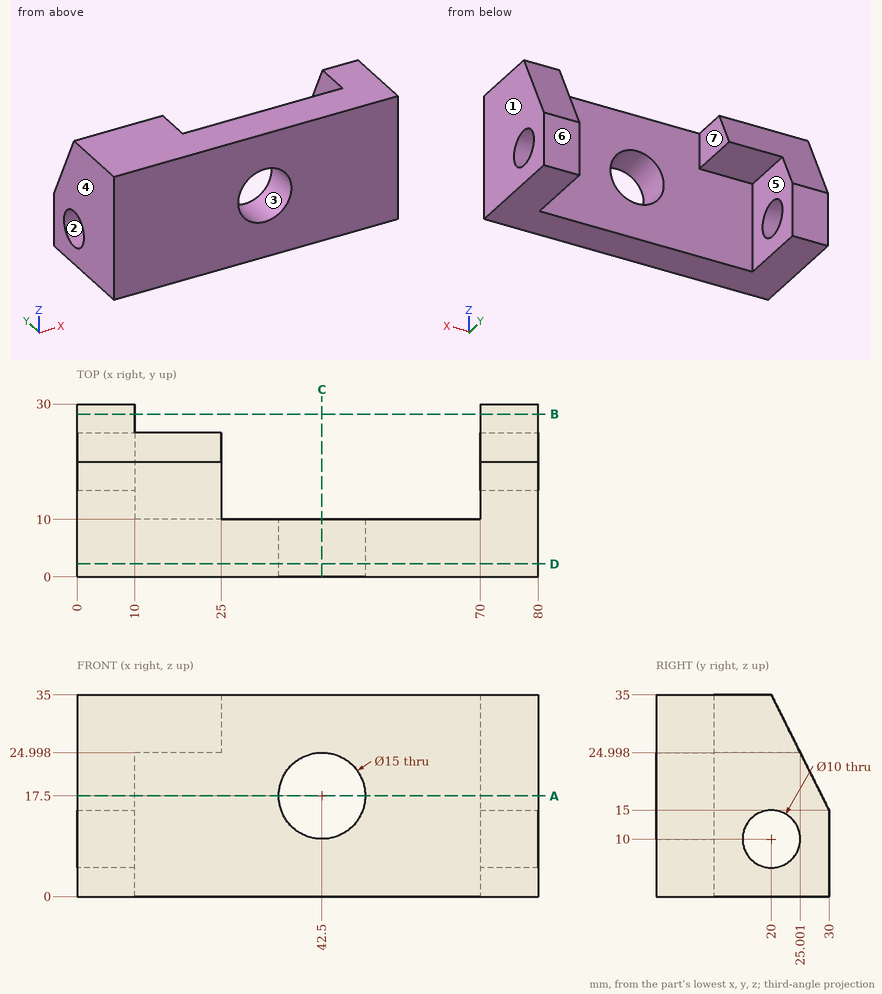
Geometry check sheet. Reference: drawing and pictorial views, mm from the part's lowest x, y, z. A direction names the side the tool comes from. Coordinates: 2 decimals unless noted, no trailing zeros. Write each loop counter-clockwise with the first axis right and the second up, starting at its lowest first coordinate (ties: lowest second). Pieces come first, ordered by that corner, then holes. Notation, with made-up numbers: (17.5, -32.5) - (42.5, -32.5) arc R8 ccw to (42.5, -22.5) - close; hole circle Ø10 at (6.25, -18.75). An arc over 180 degrees is marked (long way). Write item = value, one per line.
Q1. Cross-section at B-B (y = 28.25). Enter the section's corners in (x, z), plus the area to 3 significant figures.
Answer:
outline = (0, 0) - (10, 0) - (10, 18.5) - (0, 18.5) - close; (70, 0) - (80, 0) - (80, 18.5) - (70, 18.5) - close
area = 370 mm²
Q2. Access from +Z, -Z, +X, -X, +Y, -Y to the whole of each face (thin tool, end or side, straight path). Record for the marked faces 5, 6 and 7.
Answer:
face_5 = -Z, +Y
face_6 = +Z, -Z, +X, -X, +Y
face_7 = +Z, -Z, +Y
Q3. Mould release check, pull along X, two halves, no side actions. Record for the marked faces 1, 2, 3 and 4: released by +X, released by -X, zero draft, split by the parting line, or undercut.
Answer:
face_1 = released by +X
face_2 = zero draft
face_3 = undercut
face_4 = released by -X
Q4. Cross-section at A-A (z = 17.5). Enter the section's corners in (x, y), plus the area to 4 significant figures.
Answer:
outline = (0, 0) - (35, 0) - (35, 10) - (10, 10) - (10, 28.75) - (0, 28.75) - close; (50, 0) - (80, 0) - (80, 28.75) - (70, 28.75) - (70, 10) - (50, 10) - close
area = 1,025 mm²
Q5. Cross-section at C-C (x = 42.5). Enter the section's corners in (y, z).
Answer:
outline = (0, 0) - (10, 0) - (10, 10) - (0, 10) - close; (0, 25) - (10, 25) - (10, 35) - (0, 35) - close
Q6. Material ranges on L1, parallel to Z at x = 42.5, y = 6.75; L2, parallel to Y at x = 72.25, z = 10; L3, parallel to X at y = 2.5, z = 17.5, recorded low to high. Write a range as from..to.
Answer:
L1 = 0..10, 25..35
L2 = 0..15, 25..30
L3 = 0..35, 50..80
Q7. Cross-section at D-D (y = 2.25). Enter the section's corners in (x, z).
Answer:
outline = (0, 0) - (80, 0) - (80, 35) - (0, 35) - close; hole circle Ø15 at (42.5, 17.5)
Q8. Go/stop test with flat-tipped pins: pin 1 Ø8 at (x, z) = (10.5, 22) entering from +Y (1 decimal); pin 2 Ø10.5 at (x, z) = (30, 20.5) entering from +Y. Record where each tip stops, or that it passes through.
Answer:
pin_1 = 28.5
pin_2 = 10
